The listing builds one solid part. Answer for the finished solid, in the listing's coordinates (mm). A direction names the side the tool comes from. Round coordinates to 2 decimals unless told otherwise and drop trailing zeros. Write each loop counter-clockwise with the first axis right and the second up, starting at its lowest first coordinate (ties: lowest second). Pieces come first, ordered by that corner, then holes. Notation, with made-up numbers: (77.25, 2.25) - (105.25, 2.25) arc R17 cw to (105.25, 19.25) - close; hole circle Ø1 at (22, -40). An arc over 180 degrees is marked (long way). Return JSON: item names as keys, results as strings. Group by question number.
from build123d import *

# Parameters (mm, degrees)
SKETCH1_R           = 3.175
BOSS_EXTRUDE1_DEPTH = 7.5
SKETCH2_R           = 3.175
BOSS_EXTRUDE2_DEPTH = 7.5
BOSS_EXTRUDE3_DEPTH = 44.45
FILLET1_R           = 20
BOSS_EXTRUDE4_DEPTH = 3.75
CHAMFER1_SIZE       = 2


with BuildPart() as part:
    # Sketch1 → Boss-Extrude1 (new body)
    with BuildSketch(Plane.XY):
        with BuildLine():
            Line((-41.275, 9.525), (-0.475, 9.525))
            ThreePointArc((-0.475, 9.525), (6.596067812, 6.596067812), (9.525, -0.475))
            Line((9.525, -0.475), (9.525, -24.925))
            ThreePointArc((9.525, -24.925), (6.596067812, -31.996067812), (-0.475, -34.925))
            Line((-0.475, -34.925), (-41.275, -34.925))
            Line((-41.275, -34.925), (-41.275, 9.525))
        make_face()
        Circle(SKETCH1_R, mode=Mode.SUBTRACT)
        with Locations(Location((0, -25.4, 0), (0, 0, 180))):
            Circle(SKETCH1_R, mode=Mode.SUBTRACT)
    extrude(amount=BOSS_EXTRUDE1_DEPTH)



with BuildPart() as body_2:
    # Sketch2 → Boss-Extrude2 (new body)
    with BuildSketch(Plane.ZY.offset(41.275)):
        with BuildLine():
            Line((7.5, 9.525), (48.3, 9.525))
            ThreePointArc((48.3, 9.525), (55.371067812, 6.596067812), (58.3, -0.475))
            Line((58.3, -0.475), (58.3, -24.925))
            ThreePointArc((58.3, -24.925), (55.371067812, -31.996067812), (48.3, -34.925))
            Line((48.3, -34.925), (7.5, -34.925))
            Line((7.5, -34.925), (7.5, 9.525))
        make_face()
        with Locations(Location((48.775, 0, 0), (0, 0, 270))):
            Circle(SKETCH2_R, mode=Mode.SUBTRACT)
        with Locations(Location((48.775, -25.4, 0), (0, 0, 90))):
            Circle(SKETCH2_R, mode=Mode.SUBTRACT)
    extrude(amount=BOSS_EXTRUDE2_DEPTH)


with BuildPart() as part_1:
    add(part.part)

    add(body_2.part)  # Boss-Extrude3 merges body 2
    # Sketch3 → Boss-Extrude3 (add)
    with BuildSketch(Plane.XZ.offset(34.925)):
        with BuildLine():
            Line((-48.775, 7.5), (-41.275, 7.5))
            Line((-41.275, 7.5), (-41.275, 0))
            ThreePointArc((-41.275, 0), (-46.578300859, 2.196699141), (-48.775, 7.5))
        make_face()
    extrude(amount=-BOSS_EXTRUDE3_DEPTH)

    # Fillet1
    fillet1_edges = [part_1.edges().sort_by_distance(p)[0] for p in [
        (-41.275, -12.7, 7.5),
    ]]
    fillet(fillet1_edges, radius=FILLET1_R)

    # Sketch4 → Boss-Extrude4 (add, symmetric)
    with BuildSketch(Plane(origin=(0, -12.7, 0), x_dir=(1, 0, 0), z_dir=(0, 1, 0))):
        with BuildLine():
            Line((-0.475, -7.5), (9.525, -7.5))
            Line((9.525, -7.5), (-41.275, -58.3))
            Line((-41.275, -58.3), (-41.275, -48.3))
            Line((-41.275, -48.3), (-41.275, -27.5))
            ThreePointArc((-41.275, -27.5), (-35.417135624, -13.357864376), (-21.275, -7.5))
            Line((-21.275, -7.5), (-0.475, -7.5))
        make_face()
    extrude(amount=BOSS_EXTRUDE4_DEPTH, both=True)

    # Chamfer1
    chamfer1_edges = [part_1.edges().sort_by_distance(p)[0] for p in [
        (-3.175, 0, 7.5),
        (3.175, -25.4, 7.5),
        (-41.275, 3.175, 48.775),
        (-41.275, -28.575, 48.775),
    ]]
    chamfer(chamfer1_edges, length=CHAMFER1_SIZE)


solid = part_1.part
(1) Find section B-B (z = 6.5). Write down the section's boundary in (x, y) (3 decimals), plus the area to 3 significant figures.
(2) Find section A-A (y = -17.5). Write down the section's boundary in (x, z) (3 decimals), plus the area to 3 significant figures.
(3) Find section D-D (z = 50). State how many separate pieces and enclosed holes the cut face has, plus the area to 3 significant figures.
(4) Find section C-C (x = -27). Write down the section's boundary in (y, z) (3 decimals), plus the area to 3 significant figures.
(5) Determine the mould class of faces 4 (the flat face through (-37, 9.525, 12)), 5 (the cylindrical face through (0.41, -28.55, 2.71)), 6 (the flat face through (-15.519, -12.647, 32.544)) for opening direction X: +X half, -X half, draft (parallel to the pull), parting line (faces both ways), or undercut.
(6) For faces 1 (the flat face through (-37, -34.925, 12)), 2 (the flat face through (-41.275, 0, 43)), 3 (the flat face through (-9, -26, 7.5)), determine the directions among +Z, -Z, +X, -X, +Y, -Y from which every point of the face is accessible in a straight line to the end or side of a thin tool.
(7) Flat-ended cylindrical pins translate along their axes: pin 1 (8 mm diameter, centred on y = -15.5, z = 30.5, fed in from +X) (3 decimals); pin 2 (8.5 mm diameter, centred on x = 0, y = -25.4, fed in from +Z) (3 decimals); pin 3 (2 mm diameter, centred on x = -8.5, y = 1.5, fed in from +Z); pin 4 (5 mm diameter, centred on y = 0, z = 48.775, fed in from +X). Find the tip coordinate at first contact, or state that the pin passes through.
(8) Consider line 1 (Y direction, x = 0, z = 2.1) (3 decimals); line 2 (Z direction, x = 7.5, y = -10) (3 decimals); line 3 (X direction, y = 0.5, z = 30) (3 decimals). Determine where each line is inside the solid, lowest interval first.
Check sheet entries:
{
 "1": {"outline": "(-48.708, -34.925) - (-0.475, -34.925) arc R10 ccw to (9.525, -24.925) - (9.525, -0.475) arc R10 ccw to (-0.475, 9.525) - (-48.708, 9.525) - close; hole circle Ø8.35 at (0, -25.4); hole circle Ø8.35 at (0, 0)", "area": "2,440 mm^2"},
 "2": {"outline": "(-48.775, 7.5) arc R7.5 ccw to (-41.275, 0) - (9.525, 0) - (9.525, 7.5) - (-21.275, 7.5) arc R20 cw to (-41.275, 27.5) - (-41.275, 58.3) - (-48.775, 58.3) - close", "area": "892 mm^2"},
 "3": {"separate pieces": "3", "enclosed holes": "0", "area": "297 mm^2"},
 "4": {"outline": "(-34.925, 0) - (9.525, 0) - (9.525, 8.337) - (-8.95, 8.337) - (-8.95, 44.025) - (-16.45, 44.025) - (-16.45, 8.337) - (-34.925, 8.337) - close", "area": "638 mm^2"},
 "5": {"face 4": "draft", "face 5": "undercut", "face 6": "+X half"},
 "6": {"face 1": "+Z, -Z, +X, -X, -Y", "face 2": "+Z, +X, +Y", "face 3": "+Z, +X, -Y"},
 "7": {"pin 1": "stops at x = -9.475", "pin 2": "stops at z = 6.575", "pin 3": "stops at z = 7.5", "pin 4": "passes through"},
 "8": {"line 1": "y = -34.914 to -28.575, -22.225 to -3.175, 3.175 to 9.514", "line 2": "z = 0 to 9.525", "line 3": "x = -48.775 to -41.275"}
}
